The listing builds one solid part. Answer for the finished solid, in the listing's coordinates (mm). A direction names the side the tool comes from. Round coordinates to 2 decimals unless told otherwise and drop trailing zeros. Write each loop counter-clockwise with the first axis right and the second up, starting at its lowest first coordinate (ties: lowest second). Pieces come first, ordered by that corner, then holes. Notation, with made-up numbers: (-22.5, 50) - (-8.5, 50) arc R12 ccw to (-8.5, 64) - close; hole circle Ø11 at (58.25, 27). An arc over 180 degrees is marked (long way). Answer in a Markdown table with one row per item.
Autodesk Inventor part; units mm, degrees
ref_plane "YZ Plane" through (0, 0, 0) normal (1, 0, 0) x (0, 1, 0)
ref_plane "XZ Plane" through (0, 0, 0) normal (0, 1, 0) x (-1, 0, 0)
ref_plane "XY Plane" through (0, 0, 0) normal (0, 0, 1) x (1, 0, 0)
sketch "Esquisse1" plane through (0, 0, 0) normal (0, 0, 1) x (1, 0, 0)
  line L0 (-51.7647, 0) -> (76.2353, 0)
  line L1 (76.2353, 0) -> (76.2353, 106.1647)
  line L2 (76.2353, 106.1647) -> (-51.7647, 106.1647)
  line L3 (-51.7647, 106.1647) -> (-51.7647, 0)
  point P0 (0, 0)
  dimension "d0" = 128
extrude "Extrusion1" add sketch "Esquisse1" along normal blind 20
sketch "Esquisse2" plane through (0, 0, 20) normal (0, 0, 1) x (1, 0, 0)
  line L0 (-51.7647, 106.1647) -> (-51.7647, 0)
  line L1 (-51.7647, 61.583) -> (76.7863, 61.583)
  line L2 (76.2353, 106.1647) -> (-51.7647, 106.1647)
  arc A0 (76.2353, 61.583) -> (12.2353, 106.1647) centre (0.1874, 20.6401) ccw
  line L3 (-51.7647, 106.1647) -> (-51.7647, 61.583)
  line L4 (-51.7647, 106.1647) -> (76.2353, 106.1647)
  line L5 (76.2353, 0) -> (76.2353, 106.1647)
  line L6 (76.2353, 106.1647) -> (76.2353, 61.583)
  arc A1 (12.2353, 106.1647) -> (-51.7647, 61.583) centre (24.2774, 20.6484) ccw
  line L7 (-51.7647, 61.583) -> (-51.7647, 106.1647)
  line L8 (-51.7647, 106.1647) -> (76.2353, 106.1647)
  line L9 (76.2353, 106.1647) -> (76.2353, 61.583)
  point P0 (0, 0)
  dimension "d5" = 86.36
extrude "Extrusion2" cut sketch "Esquisse2" against normal blind 20 contours L2 A1 L0 | L2 L5 A0
sketch "Esquisse3" plane through (-51.7647, 0, 0) normal (0, -1, 0) x (1, 0, 0)
  line L0 (0, 20) -> (128, 20)
  line L1 (10, 20) -> (118, 20)
  line L2 (118, 20) -> (118, 7.5)
  line L3 (118, 7.5) -> (10, 7.5)
  line L4 (10, 7.5) -> (10, 20)
  line L5 (0, 0) -> (0, 20)
  line L6 (128, 0) -> (128, 20)
  line L7 (0, 0) -> (128, 0)
  line L8 (10, 20) -> (64, 7.5)
  line L9 (118, 20) -> (64, 7.5)
  line L10 (118, 20) -> (10, 20)
  point P0 (51.7647, 0)
  dimension "d6" = 10
  dimension "d7" = 10
  dimension "d8" = 7.5
extrude "Extrusion3" cut sketch "Esquisse3" against normal blind 60 contours L0 L9 L8
chamfer "Chanfrein1" distance 5.55 angle 45 1 edges at (12.2353, 60, 20)
fillet "Congé1" radius 10 1 edges at (12.2353, 65.55, 20)
sketch "Esquisse4" plane through (-51.7647, 0, 0) normal (0, -1, 0) x (1, 0, 0)
  line L0 (10, 12.5) -> (15, 12.5)
  line L1 (15, 12.5) -> (15, 17.5)
  line L2 (15, 17.5) -> (10, 17.5)
  line L3 (10, 17.5) -> (10, 12.5)
  line L4 (0, 20) -> (10, 20)
  line L5 (0, 0) -> (0, 20)
  point P0 (51.7647, 0)
  point P1 (5, 20)
  dimension "d15" = 5
  dimension "d16" = 5
  dimension "d17" = 2.5
  dimension "d18" = 10
extrude "Extrusion4" add sketch "Esquisse4" along normal blind 20
sketch "Esquisse5" plane through (-36.7647, 0, 17.5) normal (1, 0, 0) x (0, 0, -1)
  point P0 (17.5, 0)
sketch "Esquisse6" plane through (-36.7647, 0, 17.5) normal (1, 0, 0) x (0, 0, -1)
  line L0 (5, 0) -> (5, -20)
  line L1 (0, 0) -> (0, -20)
  line L2 (5, -20) -> (0, -20)
  line L3 (0, -20) -> (0, -10)
  line L4 (0, -10) -> (5, -10)
  line L5 (5, -10) -> (5, -20)
  point P0 (17.5, 0)
extrude "Extrusion5" add sketch "Esquisse6" along normal blind 10
sketch "Esquisse7" plane through (-51.7647, 0, 0) normal (0, -1, 0) x (1, 0, 0)
  line L0 (118, 17.5) -> (113, 17.5)
  line L1 (113, 17.5) -> (113, 12.5)
  line L2 (113, 12.5) -> (118, 12.5)
  line L3 (118, 12.5) -> (118, 17.5)
  line L4 (128, 0) -> (128, 20)
  line L5 (118, 20) -> (128, 20)
  point P0 (51.7647, 0)
  dimension "d23" = 5
  dimension "d24" = 5
  dimension "d25" = 10
  dimension "d26" = 2.5
extrude "Extrusion6" add sketch "Esquisse7" along normal blind 20
sketch "Esquisse8" plane through (66.2353, 0, 17.5) normal (1, 0, 0) x (0, 0, -1)
  line L0 (0, -20) -> (5, -20)
  line L1 (5, -10) -> (0, -10)
  line L2 (5, -20) -> (0, -20)
  line L3 (0, -20) -> (0, -10)
  line L4 (0, -10) -> (5, -10)
  line L5 (5, -10) -> (5, -20)
  point P0 (17.5, 0)
extrude "Extrusion7" add sketch "Esquisse8" along normal blind 10
properties part number "coupole"
(1) Flat-ended cylindrical pins translate along their axes: pin 1 (2.5 mm diameter, centred on x = -34, z = 14, fed in from +Y); pin 2 (5.5 mm diameter, centred on y = -4, z = 14.5, fed in from +X); pin 3 (2 mm diameter, centred on x = 31, y = 34, fed in from +Z); pin 4 (7.5 mm diameter, centred on x = -31, y = -6, fed in from -Z). Find the tip coordinate at first contact, or state that the pin passes through.
Checked values:
| item | result |
|---|---|
| pin 1 | stops at y = 85.5 |
| pin 2 | stops at x = 66.24 |
| pin 3 | stops at z = 12.08 |
| pin 4 | passes through |
(2) For a pull along X with two mould halves and no side action, classify faces 1 (the flat face through (67, -12, 17.5)), 2 (the cylindrical face through (-24.62, 91.83, 10.14)), 3 (the flat face through (-36.765, -5, 15)) as pulls with the +X half, pulls with the -X half, needs draft (parallel to the pull), parting line crosses it, or undercut.
Checked values:
| item | result |
|---|---|
| face 1 | needs draft |
| face 2 | pulls with the -X half |
| face 3 | undercut |
(3) Section A-A (x = -34) is taken. Give the vertices of the cut face in (y, z).
Checked values:
| item | result |
|---|---|
| outline | (-20, 12.5) - (-10, 12.5) - (-10, 17.5) - (-20, 17.5) - close; (0, 0) - (84.38, 0) - (84.38, 20) - (69.69, 20) arc R10 ccw to (63.97, 18.2) - (0, 18.2) - close |
(4) Section D-D (x = 56.5) is taken. Give the vertices of the cut face in (y, z), and give its area (3 significant figures).
Checked values:
| item | result |
|---|---|
| outline | (0, 0) - (86.13, 0) - (86.13, 20) - (69.69, 20) arc R10 ccw to (63.37, 17.75) - (0, 17.75) - close |
| area | 1,580 mm2 |
(5) Section C-C (z = 4.25) is taken. Give the vertices of the cut face in (x, y).
Checked values:
| item | result |
|---|---|
| outline | (-51.76, 0) - (76.24, 0) - (76.24, 61.58) arc R86.37 ccw to (12.24, 106.16) arc R86.36 ccw to (-51.76, 61.58) - close |
(6) Section B-B (y = 67) is taken. Give the vertices of the cut face in (x, z).
Checked values:
| item | result |
|---|---|
| outline | (-48.59, 0) - (73.06, 0) - (73.06, 20) - (66.24, 20) - (64.64, 19.63) - (-40.17, 19.63) - (-41.76, 20) - (-48.59, 20) - close |
(7) Find the intervals of material crossed by line 1 (Y direction, x = 7, z = 3.75); line 2 (Z direction, x = -27, y = 11); line 3 (X direction, y = 93, z = 2.5), in increasing order.
Checked values:
| item | result |
|---|---|
| line 1 | y = 0 to 105.26 |
| line 2 | z = 0 to 16.58 |
| line 3 | x = -22.87 to 47.34 |
(8) For faces 4 (the flat face through (67, -12, 12.5)), 5 (the flat face through (71, -10, 15)), 6 (the flat face through (-32, -10, 15)), 7 (the flat face through (39.613, 34.358, 13.838)), 8 (the flat face through (-26.765, -15, 15)), determine the directions among +Z, -Z, +X, -X, +Y, -Y from which every point of the face is accessible in a straight line to the end or side of a thin tool.
Checked values:
| item | result |
|---|---|
| face 4 | -Z, +X, -X, -Y |
| face 5 | +Z, -Z, +X |
| face 6 | +Z, -Z |
| face 7 | +Z, -Y |
| face 8 | +Z, -Z, -Y |
